from build123d import *

# Parameters (mm, degrees)
F0_W          = 1.27
F0_H          = 20.32
F1_DEPTH      = 2.54
F1_DEPTH_BACK = 2.54
F2_R          = 1.26999
F3_R          = 0.635
F4_DEPTH      = 5.08


# Not quite as in the source:
# - a fillet or chamfer is up to 0.001 mm smaller than in the source, because OpenCascade refuses the exact size


with BuildPart() as f1:
    # F0 (on Top) → F1 (new body, two sides)
    with BuildSketch(Plane.XY) as f1_sk:
        with Locations((0.635, -0.508000601)):
            Rectangle(F0_W, F0_H)
    extrude(amount=F1_DEPTH)
    extrude(f1_sk.sketch, amount=-F1_DEPTH_BACK)

    # F2 (radius 1.27 in the source; OpenCascade refuses exactly that, so slightly less here)
    f2_edges = [f1.edges().sort_by_distance(p)[0] for p in [
        (1.27, 9.651999, 0),
        (1.27, -0.508001, 2.54),
        (1.27, -0.508001, -2.54),
        (1.27, -10.668001, 0),
    ]]
    fillet(f2_edges, radius=F2_R)

    # F3 (on face) → F4 (join)
    with BuildSketch(Plane(origin=(0, 0, 0), x_dir=(0, -1, 0), z_dir=(-1, 0, 0))):
        Circle(F3_R)
    extrude(amount=F4_DEPTH)


solid = f1.part
Design review of the part built by this model. Coordinates are the model's own, in mm. A direction names the side the tool comes from. Coordinates: 2 decimals unless noted, no trailing zeros. Order: outer loops, then holes, each group sorted by start corner. A loop starts at its lowest first (then second) coordinate and runs counter-clockwise, first axis right, second up.
Item 1: For faces 1 (the flat face through (-5.08, 0, 0)), 2 (the cylindrical face through (-2.5, 0.08, 0.63)), list the 3-axis set-ups (+Z, -Z, +X, -X, +Y, -Y) from which the entire face can be reached by the end or side of a thin tool; tool diameter is ignored.
Item 2: For line 1 (X direction, y = 4, z = -0.85); line 2 (X direction, y = 4, z = 1.5); line 3 (Y direction, x = -2.75, z = 0.3), list the stretches that pass through material, from the lowest coordinate up.
Item 3: Take a section at D-D, the plane x = -4.5. Write out the cut boundary in (y, z) (3 decimals).
Item 4: For pin 1 Ø1.5 at (y, z) = (-4, -0.5) entering from -X, flat-tipped, find the tip position at first contact; note if it passes through.
The answers:
1. face 1: +Z, -Z, -X, +Y, -Y
1. face 2: -X
2. line 1: x = 0 to 1.27
2. line 2: x = 0 to 1.25
2. line 3: y = -0.56 to 0.56
3. outline: circle Ø1.27 at (0, 0)
4. pin 1: stops at x = 0
